Here's how the part is built. I have some questions about the finished solid (model axes, mm). Coordinates: 2 decimals unless noted, no trailing zeros. Order: outer loops, then holes, each group sorted by start corner. A loop starts at its lowest first (then second) coordinate and runs counter-clockwise, first axis right, second up. Notation, with made-up numbers: (55, -16) - (89, -16) arc R21 ccw to (89, 23) - close; hole circle Ø3 at (88.25, -34). An arc over 180 degrees is marked (long way). Use one line per item in the form item = value. Start each with the question number.
from build123d import *

# Parameters (mm, degrees)
BOSS_EXTRUDE1_DEPTH = 10


with BuildPart() as part:
    # Sketch1 → Boss-Extrude1 (new body)
    with BuildSketch(Plane(origin=(0, 0, 0), x_dir=(0, 0, -1), z_dir=(1, 0, 0))):
        with BuildLine():
            Line((0, 6.825), (0, 0))
            Line((0, 0), (18, 0))
            Line((18, 0), (9, 20))
            Line((9, 20), (0, 20))
            Line((0, 20), (0, 13.175))
            ThreePointArc((0, 13.175), (2.24506403, 12.24506403), (3.175, 10))
            ThreePointArc((3.175, 10), (2.24506403, 7.75493597), (0, 6.825))
        make_face()
        with BuildLine():
            Line((-18, 0), (0, 0))
            Line((0, 0), (0, 6.825))
            ThreePointArc((0, 6.825), (-3.175, 10), (0, 13.175))
            Line((0, 13.175), (0, 20))
            Line((0, 20), (-9, 20))
            Line((-9, 20), (-18, 0))
        make_face()
    extrude(amount=BOSS_EXTRUDE1_DEPTH)


solid = part.part
1) Suppose I cut it at C-C, the plane z = 1. List the corners of the cut face in (x, y) for me, then the cut area to 3 significant figures.
2) Suppose I cut it at B-B, the plane x = 6. List the corners of the cut face in (y, z) for me (3 decimals), then the cut area to 3 significant figures.
3) For pin 1 (4 mm diameter, centred on x = 5, y = 8.5, fed in from -Z) (3 decimals); pin 2 (5 mm diameter, centred on x = 8.5, z = 14, fed in from +Y); pin 3 (4 mm diameter, centred on x = 6.5, y = 6.5, fed in from -Z) (3 decimals), each with a flat end and sliding along its axis, tell me the tip position at first contact or that it passes through.
4) Suppose I cut it at A-A, the plane y = 11. List the corners of the cut face in (x, z) for me.
5) I need wall thicknesses on probe 1 along Z at (x, y) = (3.5, 7.5) (3 decimals); probe 2 along Z at (x, y) = (5.75, 11); probe 3 along Z at (x, y) = (4, 3.5) (3 decimals). Which ranges of each line are inside material? Lowest first, please. Write a range as [from, to].
6) Suppose I cut it at D-D, the plane y = 17. List the corners of the cut face in (x, z) for me, then the cut area to 3 significant figures.
From the geometry:
q1.outline = (0, 0) - (10, 0) - (10, 6.99) - (0, 6.99) - close; (0, 13.01) - (10, 13.01) - (10, 20) - (0, 20) - close
q1.area = 140 mm2
q2.outline = (0, -18) - (20, -9) - (20, 9) - (0, 18) - close; hole circle Ø6.35 at (10, 0)
q2.area = 508 mm2
q3.pin_1 = -15.075
q3.pin_2 = 14.44
q3.pin_3 = -15.975
q4.outline = (0, -13.05) - (10, -13.05) - (10, -3.01) - (0, -3.01) - close; (0, 3.01) - (10, 3.01) - (10, 13.05) - (0, 13.05) - close
q5.probe_1 = [-14.625, -1.957], [1.957, 14.625]
q5.probe_2 = [-13.05, -3.01], [3.01, 13.05]
q5.probe_3 = [-16.425, 16.425]
q6.outline = (0, -10.35) - (10, -10.35) - (10, 10.35) - (0, 10.35) - close
q6.area = 207 mm2
